Design review of the part shown in the three views and the two pictorial views. Dimensions are in mm from the part's minimum x, y and z. A direction names the side the tool comes from. Give positions to 0.01 mm unless a question says otherwise; leave off trailing zeros. Order: outer loops, then holes, each group sorted by start corner. A loop starts at its lowest first (then second) coordinate and runs counter-clockwise, first axis right, second up.
Item 1: Consider section C-C (y = 16.5). Give the boundary of the cut face in (x, z).
Item 2: For probe 1 along Y at (x, z) = (10, 0.8); probe 2 along Y at (x, z) = (33, 0.75) (1 decimal); probe 3 along X at (y, z) = (2.5, 0.7), list the stretches that pass through material, from the lowest coordinate up.
Item 3: Machinability: for the marked faces 4, 5 and 6, which of the approach directions +Z, -Z, +X, -X, +Y, -Y give a long, thin tool a straight path to every point of the face, cutting with its end or side? Answer none if there is none.
Item 4: The part is to be moulded in two halves that separate along Y. For the marked faces 1, 2 and 3, say which applies: released by +Y, released by -Y, zero draft, split by the parting line, or undercut.
Item 5: Consider section A-A (z = 0.4). Give the boundary of the cut face in (x, y), plus the area to 3 significant figures.
Item 6: Consider section B-B (x = 13.5). Give the boundary of the cut face in (y, z), plus the area to 3 significant figures.
Item 7: For P1, Ø1.5, axis at y = 2.5, z = 1.5, coming from the +X side; P2, Ø0.9, axis at x = 37.5, z = 2, coming from the -Y side, all flat-tipped, find the tip position at first contact; note any pin that passes through.
Item 8: Consider section D-D (y = 4.5). Give the boundary of the cut face in (x, z).
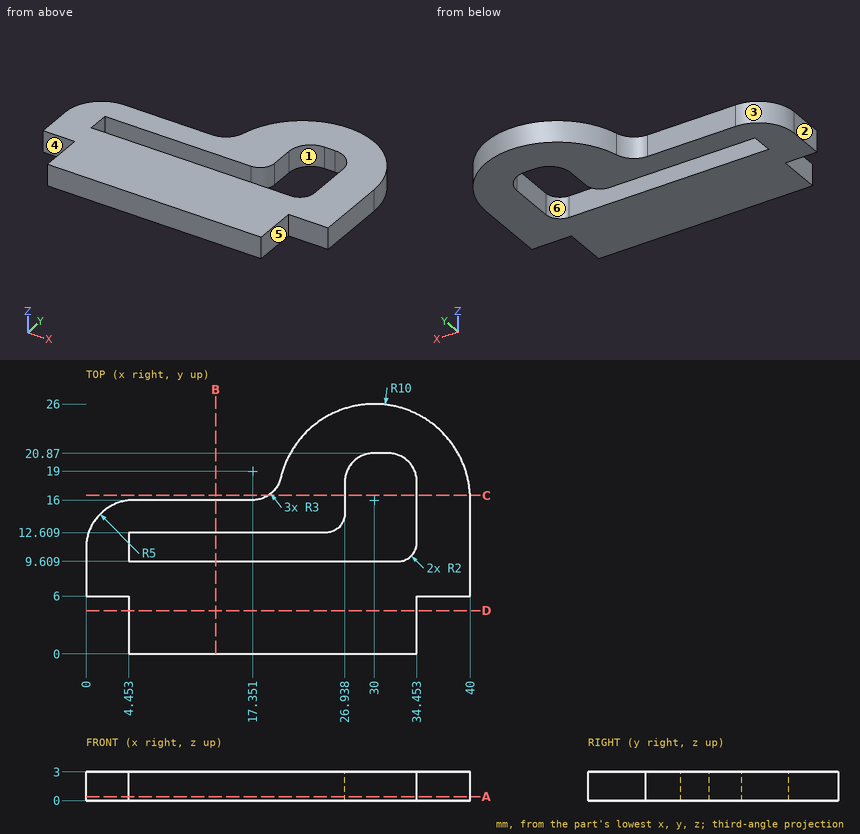
Resolved:
1. outline: (19.01, 0) - (26.94, 0) - (26.94, 3) - (19.01, 3) - close; (34.45, 0) - (39.99, 0) - (39.99, 3) - (34.45, 3) - close
2. probe 1: y = 0 to 9.61, 12.61 to 16
2. probe 2: y = 0 to 9.7, 20.4 to 25.5
2. probe 3: x = 4.45 to 34.45
3. face 4: +Z, -Z, -X, -Y
3. face 5: +Z, -Z, +X, -Y
3. face 6: +Z, -Z
4. face 1: undercut
4. face 2: zero draft
4. face 3: released by +Y
5. outline: (0, 6) - (4.45, 6) - (4.45, 0) - (34.45, 0) - (34.45, 6) - (40, 6) - (40, 16) arc R10 ccw to (20.27, 18.31) arc R3 cw to (17.35, 16) - (5, 16) arc R5 ccw to (0, 11) - close; hole (4.45, 9.61) - (32.45, 9.61) arc R2 ccw to (34.45, 11.61) - (34.45, 17.87) arc R3 ccw to (31.45, 20.87) - (29.94, 20.87) arc R3 ccw to (26.94, 17.87) - (26.94, 14.61) arc R2 cw to (24.94, 12.61) - (4.45, 12.61) - close
5. area: 585 mm2
6. outline: (0, 0) - (9.61, 0) - (9.61, 3) - (0, 3) - close; (12.61, 0) - (16, 0) - (16, 3) - (12.61, 3) - close
6. area: 39.0 mm2
7. P1: stops at x = 34.45
7. P2: stops at y = 6
8. outline: (4.45, 0) - (34.45, 0) - (34.45, 3) - (4.45, 3) - close
